CAD build for the part. Positions are in the model's coordinates, mm. A direction names the side the tool comes from. Give positions to 0.01 mm unless a question says otherwise; leave off trailing zeros. Loops run counter-clockwise (first coordinate to the right, second up) from the corner with the lowest first, then second, coordinate; pieces in that order, holes last. Notation, with made-up numbers: M 67,78.25 L 99,78.25 A19 ccw 99,107.25 Z; hole C 75,-15.5 d7. An arc over 180 degrees is marked long. Answer as CSV lines item,"result".
from build123d import *
from build123d.topology import SkipClean

# Parameters (mm, degrees)
SKETCH1_R                = 3.175
BOSS_EXTRUDE1_DEPTH      = 18
CUT_EXTRUDE4_DEPTH       = 3.5
CUT_EXTRUDE4_DEPTH_BACK  = 3.5
CUT_EXTRUDE5_DEPTH       = 6.5
SKETCH9_W                = 50
SKETCH9_H                = 5
BOSS_EXTRUDE2_DEPTH      = 15.5
FILLET8_R                = 2.5
BOSS_EXTRUDE3_REACH      = 75.76
SKETCH13_W               = 5
SKETCH13_H               = 15.14
SKETCH16_W               = 15.5
SKETCH16_H               = 5
BOSS_EXTRUDE4_DEPTH      = 15.14
CUT_EXTRUDE8_REACH       = 77.34
CUT_EXTRUDE9_DEPTH       = 5.5
CUT_EXTRUDE10_DEPTH      = 1
CUT_EXTRUDE11_START      = -1
SKETCH20_R               = 5
CUT_EXTRUDE11_DEPTH      = 1
SKETCH21_W               = 31
SKETCH21_H               = 15.05
CUT_EXTRUDE12_DEPTH      = 5
BOSS_EXTRUDE11_DEPTH     = 20.14
SKETCH31_R               = 2.125
CUT_EXTRUDE16_DEPTH      = 20.14
SKETCH38_R               = 3.25
CUT_EXTRUDE19_DEPTH      = 8
CUT_EXTRUDE21_DEPTH      = 3
CUT_EXTRUDE21_DEPTH_BACK = 1
SKETCH39_R               = 2.625
M5_CUT_DEPTH             = 9.14


with BuildPart() as part:
    # Sketch1 → Boss-Extrude1 (new body)
    with BuildSketch(Plane(origin=(0, 0, 0), x_dir=(0, 0, -1), z_dir=(1, 0, 0))):
        with BuildLine():
            Line((-64.5, -12.57), (-14.5, -12.57))
            ThreePointArc((-14.5, -12.57), (-7.668930825, -8.855100607), (0, -7.57))
            ThreePointArc((0, -7.57), (6.813585795, 3.298476711), (-5.937768577, 4.695508953))
            ThreePointArc((-5.937768577, 4.695508953), (-9.447591416, 2.520990205), (-13.536399337, 3.094608482))
            Line((-13.536399337, 3.094608482), (-15.082858667, 4.641067812))
            ThreePointArc((-15.082858667, 4.641067812), (-18.327092155, 6.808795325), (-22.153926479, 7.57))
            Line((-22.153926479, 7.57), (-24.481144331, 7.57))
            Line((-24.481144331, 7.57), (-64.5, 7.57))
            Line((-64.5, 7.57), (-64.5, -12.57))
        make_face()
        Circle(SKETCH1_R, mode=Mode.SUBTRACT)
        with BuildLine():
            Line((-52, 3.175), (-40, 3.175))
            ThreePointArc((-40, 3.175), (-36.825, 0), (-40, -3.175))
            Line((-40, -3.175), (-52, -3.175))
            ThreePointArc((-52, -3.175), (-55.175, 0), (-52, 3.175))
        make_face(mode=Mode.SUBTRACT)
    extrude(amount=BOSS_EXTRUDE1_DEPTH)

    # Sketch7 → Cut-Extrude4 (cut, two sides: drawn at the far end of the back side and taken through both)
    with BuildSketch(Plane.ZY.offset(-9).offset(-CUT_EXTRUDE4_DEPTH_BACK)):
        with BuildLine():
            Line((68.683555498, -7.57), (38.854158917, -7.57))
            ThreePointArc((38.854158917, -7.57), (29.611049041, -2.529814803), (26.6391325, 7.57))
            Line((26.6391325, 7.57), (68.683555498, 7.57))
            Line((68.683555498, 7.57), (68.683555498, -7.57))
        make_face()
    extrude(amount=CUT_EXTRUDE4_DEPTH + CUT_EXTRUDE4_DEPTH_BACK, mode=Mode.SUBTRACT)

    # Sketch8 → Cut-Extrude5 (cut)
    with BuildSketch(Plane(origin=(18, 0, 0), x_dir=(0, 0, -1), z_dir=(1, 0, 0))):
        Polygon((-14.5, -12.57), (-14.5, -7.57), (-22.153926479, 7.57), (4.247659324, 15.20685859), (9.411129334, 3.26000641), (7.386239134, -6.35822204), align=None)
    cut_extrude5 = extrude(amount=-CUT_EXTRUDE5_DEPTH, mode=Mode.SUBTRACT)

    # Sketch9 → Boss-Extrude2 (add)
    with BuildSketch(Plane.ZY):
        with Locations((39.5, -10.07)):
            Rectangle(SKETCH9_W, SKETCH9_H)
    extrude(amount=BOSS_EXTRUDE2_DEPTH)

    # Mirror2: Cut-Extrude5 across plane
    add(cut_extrude5.mirror(Plane.ZY.offset(-9)), mode=Mode.SUBTRACT)

    # Fillet8
    fillet8_edges = [part.edges().sort_by_distance(p)[0] for p in [
        (3.25, 7.57, 22.153926479),
        (14.75, 7.57, 22.153926479),
        (14.75, -7.57, 14.5),
    ]]
    fillet(fillet8_edges, radius=FILLET8_R)

    # Boss-Extrude3: up to this face of the body (flat: up to its plane)
    boss_extrude3_end = Plane(part.part.faces().sort_by_distance((-15.5, -10.07, 39.5))[0])
    # Sketch13 → Boss-Extrude3 (add, up to the picked face)
    with BuildSketch(Plane(origin=(18, 0, 0), x_dir=(0, 0, -1), z_dir=(1, 0, 0)), mode=Mode.PRIVATE) as boss_extrude3_sk1:
        with Locations((-62, 0)):
            Rectangle(SKETCH13_W, SKETCH13_H)
    boss_extrude3_tool1 = split(extrude(boss_extrude3_sk1.sketch, amount=-BOSS_EXTRUDE3_REACH, mode=Mode.PRIVATE), bisect_by=boss_extrude3_end, keep=Keep.BOTH, mode=Mode.PRIVATE)
    add(boss_extrude3_tool1.solids().sort_by(Axis((18, 0, 62), (-1, 0, 0)))[0])

    # Sketch16 → Boss-Extrude4 (add)
    with BuildSketch(Plane(origin=(0, -7.57, 0), x_dir=(1, 0, 0), z_dir=(0, 1, 0))):
        with Locations((-7.75, -32.05)):
            Rectangle(SKETCH16_W, SKETCH16_H)
    extrude(amount=BOSS_EXTRUDE4_DEPTH)

    # Cut-Extrude8: up to this face of the body (flat: up to its plane)
    cut_extrude8_end = Plane(part.part.faces().sort_by_distance((-7.75, 0, 29.55))[0])
    # Sketch14 → Cut-Extrude8 (cut, up to the picked face)
    with BuildSketch(Plane.XY.offset(64.5), mode=Mode.PRIVATE) as cut_extrude8_sk1:
        with BuildLine():
            Line((-15.5, 3.175), (-15.5, -3.175))
            ThreePointArc((-15.5, -3.175), (-12.325, 0), (-15.5, 3.175))
        make_face()
    cut_extrude8_tool1 = split(extrude(cut_extrude8_sk1.sketch, amount=-CUT_EXTRUDE8_REACH, mode=Mode.PRIVATE), bisect_by=cut_extrude8_end, keep=Keep.BOTH, mode=Mode.PRIVATE)
    add(cut_extrude8_tool1.solids().sort_by(Axis((-14.152488, 0, 64.5), (0, 0, -1)))[0], mode=Mode.SUBTRACT)

    # Sketch17 → Cut-Extrude9 (cut)
    with BuildSketch(Plane(origin=(18, 0, 0), x_dir=(0, 0, -1), z_dir=(1, 0, 0))):
        with BuildLine():
            Line((-40, -4.375), (-52, -4.375))
            ThreePointArc((-52, -4.375), (-56.375, 0), (-52, 4.375))
            Line((-52, 4.375), (-40, 4.375))
            ThreePointArc((-40, 4.375), (-35.625, 0), (-40, -4.375))
        make_face()
    extrude(amount=-CUT_EXTRUDE9_DEPTH, mode=Mode.SUBTRACT)

    # Sketch19 → Cut-Extrude10 (cut)
    with BuildSketch(Plane.XY.offset(64.5)):
        with BuildLine():
            Line((-15.5, 5), (-15.5, -5))
            ThreePointArc((-15.5, -5), (-10.5, 0), (-15.5, 5))
        make_face()
    extrude(amount=-CUT_EXTRUDE10_DEPTH, mode=Mode.SUBTRACT)

    # Sketch20 → Cut-Extrude11 (cut)
    with BuildSketch(Plane(origin=(0, 0, 29.55), x_dir=(-1, 0, 0), z_dir=(0, 0, -1)).offset(CUT_EXTRUDE11_START)):
        with Locations((15.5, 0)):
            Circle(SKETCH20_R)
    extrude(amount=CUT_EXTRUDE11_DEPTH, mode=Mode.SUBTRACT)

    # Mirror3: part across plane


with BuildPart() as part_1:
    with SkipClean():  # the faces are left unmerged after this step: merging them gives an invalid solid
        add(part.part)
        add(part.part.mirror(Plane(origin=(-15.5, 0, 0), x_dir=(0, 0, 1), z_dir=(1, 0, 0))))

    # Sketch21 → Cut-Extrude12 (cut)
    with SkipClean():  # the faces are left unmerged after this step: merging them gives an invalid solid
        with BuildSketch(Plane(origin=(0, -7.57, 0), x_dir=(1, 0, 0), z_dir=(0, 1, 0))):
            with Locations((-15.5, -22.025)):
                Rectangle(SKETCH21_W, SKETCH21_H)
        extrude(amount=-CUT_EXTRUDE12_DEPTH, mode=Mode.SUBTRACT)

    # Sketch30 → Boss-Extrude11 (add)
    with SkipClean():  # the faces are left unmerged after this step: merging them gives an invalid solid
        with BuildSketch(Plane(origin=(0, 7.57, 0), x_dir=(1, 0, 0), z_dir=(0, 1, 0))):
            with BuildLine():
                Line((0, -24.675), (0, -27.425))
                ThreePointArc((0, -27.425), (-1.50260191, -28.04739809), (-2.125, -29.55))
                Line((-2.125, -29.55), (-4.875, -29.55))
                ThreePointArc((-4.875, -29.55), (-3.447145558, -26.102854442), (0, -24.675))
            make_face()
            with BuildLine():
                Line((11, -64.5), (8.25, -64.5))
                ThreePointArc((8.25, -64.5), (13.125, -69.375), (18, -64.5))
                Line((18, -64.5), (15.25, -64.5))
                ThreePointArc((15.25, -64.5), (13.125, -66.625), (11, -64.5))
            make_face()
            with BuildLine():
                Line((-42, -64.5), (-39.25, -64.5))
                ThreePointArc((-39.25, -64.5), (-44.125, -69.375), (-49, -64.5))
                Line((-49, -64.5), (-46.25, -64.5))
                ThreePointArc((-46.25, -64.5), (-44.125, -66.625), (-42, -64.5))
            make_face()
        boss_extrude11 = extrude(amount=-BOSS_EXTRUDE11_DEPTH)

    # Sketch31 → Cut-Extrude16 (cut)
    with SkipClean():  # the faces are left unmerged after this step: merging them gives an invalid solid
        with BuildSketch(Plane(origin=(0, 7.57, 0), x_dir=(1, 0, 0), z_dir=(0, 1, 0))):
            with Locations(Location((0, -29.55, 0), (0, 0, 270))):
                Circle(SKETCH31_R)
            with Locations(Location((13.125, -64.5, 0), (0, 0, 270))):
                Circle(SKETCH31_R)
            with Locations(Location((-44.125, -64.5, 0), (0, 0, 270))):
                Circle(SKETCH31_R)
        cut_extrude16 = extrude(amount=-CUT_EXTRUDE16_DEPTH, mode=Mode.SUBTRACT)

    # Mirror4: Boss-Extrude11, Cut-Extrude16 across plane
    with SkipClean():  # the faces are left unmerged after this step: merging them gives an invalid solid
        add(boss_extrude11.mirror(Plane(origin=(-15.5, 0, 0), x_dir=(0, 0, 1), z_dir=(1, 0, 0))))
        add(cut_extrude16.mirror(Plane(origin=(-15.5, 0, 0), x_dir=(0, 0, 1), z_dir=(1, 0, 0))), mode=Mode.SUBTRACT)

    # Sketch38 → Cut-Extrude19 (cut)
    with SkipClean():  # the faces are left unmerged after this step: merging them gives an invalid solid
        with BuildSketch(Plane.XZ.offset(12.57)):
            with Locations(Location((-31, 29.55, 0), (0, 0, 270))):
                Circle(SKETCH38_R)
            with Locations(Location((0, 29.55, 0), (0, 0, 270))):
                Circle(SKETCH38_R)
            with Locations(Location((13.125, 64.5, 0), (0, 0, 270))):
                Circle(SKETCH38_R)
            with Locations(Location((-44.125, 64.5, 0), (0, 0, 270))):
                Circle(SKETCH38_R)
        extrude(amount=-CUT_EXTRUDE19_DEPTH, mode=Mode.SUBTRACT)

    # Sketch32 → Cut-Extrude21 (cut, two sides: drawn at the far end of the back side and taken through both)
    with SkipClean():  # the faces are left unmerged after this step: merging them gives an invalid solid
        with BuildSketch(Plane.XZ.offset(2.57).offset(-CUT_EXTRUDE21_DEPTH_BACK)):
            Polygon((-26.154818283, 22.133830878), (-22.154818283, 29.062034108), (-31, 34.168802154), (-35, 31.859401077), (-35, 27.240598923), align=None)
            Polygon((11.929566037, 60.038579713), (8.663579713, 63.304566037), (2.173721464, 69.777896049), (7.838839832, 75.443014417), (14.320433963, 68.961420287), (17.586420287, 65.695433963), (16.390986324, 61.234013676), align=None)
            Polygon((-45.320433963, 68.961420287), (-48.586420287, 65.695433963), (-47.390986324, 61.234013676), (-42.929566037, 60.038579713), (-39.663579713, 63.304566037), (-33.173721464, 69.777896049), (-38.838839832, 75.443014417), align=None)
            Polygon((4, 27.240598923), (-4.845181717, 22.133830878), (-8.845181717, 29.062034108), (0, 34.168802154), (4, 31.859401077), align=None)
        extrude(amount=CUT_EXTRUDE21_DEPTH + CUT_EXTRUDE21_DEPTH_BACK, mode=Mode.SUBTRACT)

    # Sketch39 → M5_Cut (cut)
    with SkipClean():  # the faces are left unmerged after this step: merging them gives an invalid solid
        with BuildSketch(Plane(origin=(0, 7.57, 0), x_dir=(1, 0, 0), z_dir=(0, 1, 0))):
            with Locations(Location((-31, -29.55, 0), (0, 0, 270))):
                Circle(SKETCH39_R)
            with Locations(Location((0, -29.55, 0), (0, 0, 270))):
                Circle(SKETCH39_R)
            with Locations(Location((13.125, -64.5, 0), (0, 0, 270))):
                Circle(SKETCH39_R)
            with Locations(Location((-44.125, -64.5, 0), (0, 0, 270))):
                Circle(SKETCH39_R)
        extrude(amount=-M5_CUT_DEPTH, mode=Mode.SUBTRACT)


solid = part_1.part
1) Drill centre lines: line 1 (X direction, y = -6.5, z = 54); line 2 (Z direction, x = -14.5, y = -5.25); line 3 (X direction, y = -10.75, z = 12.5). Where is each one in solid material? Low to high. Write a range as from..to.
Answer below:
line 1,"x = -49..-43.5, -36.5..-31, 0..5.5, 12.5..18"
line 2,"z = 29.55..34.55, 59.5..64.5"
line 3,"x = -42.5..-37.5, 6.5..11.5"
2) Band-saw the part on A-A on y = 1.25. Give the number of separate pieces and of enclosed holes in the cut face, and give its area (3 significant figures).
Answer below:
separate pieces,"6"
enclosed holes,"4"
area,"1,250 mm^2"
3) Which spindle directions (+Z, -Z, +X, -X, +Y, -Y) get a long thin tool onto all of the face, cutting with end or side? Do faces 4 (the face through (3, -3.175, 46)), 5 (the face through (-36.5, 3.5, 43.3)), 6 (the face through (-31, -5, 21)), 7 (the face through (11, -1.57, 67)). Say none if no direction does.
Answer below:
face 4,"+X, -X"
face 5,"+Y"
face 6,"-Z, +Y, -Y"
face 7,"none"
4) Mould opens along Y. For faces 1 (the face through (-40, -7.57, 49)), 2 (the face through (-32.82, -3.54, 25.98)), 3 (the face through (-40, -8.9, 7.8)) say: +Y half, -Y half, draft (parallel to the pull), parting line (faces both ways), or undercut.
Answer below:
face 1,"+Y half"
face 2,"undercut"
face 3,"-Y half"
5) Band-saw the part on B-B on x = -24.5. Give the cut face in (y, z), and give its area (3 significant figures).
Answer below:
outline,"M -12.57,29.55 L -5.57,29.55 L -5.57,30.42 L -1.57,30.42 L -1.57,29.55 L 7.57,29.55 L 7.57,34.55 L -7.57,34.55 L -7.57,59.5 L 7.57,59.5 L 7.57,64.5 L -12.57,64.5 Z"
area,"323 mm^2"
6) Flat gauge pins, fed straight in: pin 1 (7.5 mm diameter, centred on y = -1, z = 50, fed in from -X); pin 2 (10 mm diameter, centred on y = -2.5, z = 9.5, fed in from +X); pin 3 (3 mm diameter, centred on x = -2, y = 3, fed in from +Z); pin 4 (12 mm diameter, centred on x = -24, z = 45.5, fed in from +Y). Where does each tip first touch, or does it go through?
Answer below:
pin 1,"stops at x = -49"
pin 2,"stops at x = 11.5"
pin 3,"stops at z = 64.5"
pin 4,"stops at y = -7.57"
